from build123d import *

# Parameters (mm, degrees)
SKETCH2_W           = 33
SKETCH2_H           = 28
BOSS_EXTRUDE1_DEPTH = 46
CUT_EXTRUDE2_DEPTH  = 59.318093247
CUT_EXTRUDE4_START  = -3
CUT_EXTRUDE4_DEPTH  = 27
FILLET2_R           = 12.5
FILLET3_R           = 12.5
FILLET4_R           = 6
SKETCH7_W           = 13
SKETCH7_H           = 23
CUT_EXTRUDE5_DEPTH  = 9
SKETCH8_R           = 6.5
CUT_EXTRUDE6_DEPTH  = 9
SKETCH9_R           = 1
CUT_EXTRUDE7_DEPTH  = 9
SKETCH10_R          = 2.5
SKETCH10_R_2        = 1.3
CUT_EXTRUDE8_DEPTH  = 9


with BuildPart() as part:
    # Sketch2 → Boss-Extrude1 (new body)
    with BuildSketch(Plane.XY):
        Rectangle(SKETCH2_W, SKETCH2_H)
    extrude(amount=BOSS_EXTRUDE1_DEPTH)

    # Sketch5 → Cut-Extrude2 (cut, through all)
    with BuildSketch(Plane(origin=(16.5, 0, 0), x_dir=(0, 0, -1), z_dir=(1, 0, 0))):
        Polygon((-5, -14), (-46, 2), (-46, -14), align=None)
    extrude(amount=-CUT_EXTRUDE2_DEPTH, mode=Mode.SUBTRACT)

    # Sketch6 → Cut-Extrude4 (cut)
    with BuildSketch(Plane(origin=(16.5, 0, 0), x_dir=(0, 0, -1), z_dir=(1, 0, 0)).offset(CUT_EXTRUDE4_START)):
        Polygon((-5, -14), (-2.5, -14), (-2.5, 3.5), (-40.5, 3.5), (-40.5, -0.146341463), align=None)
    extrude(amount=-CUT_EXTRUDE4_DEPTH, mode=Mode.SUBTRACT)

    # Fillet2
    fillet2_edges = [part.edges().sort_by_distance(p)[0] for p in [
        (-13.5, 1.676829268, 40.5),
        (13.5, 1.676829268, 40.5),
    ]]
    fillet(fillet2_edges, radius=FILLET2_R)

    # Fillet3
    fillet3_edges = [part.edges().sort_by_distance(p)[0] for p in [
        (-16.5, 8, 46),
        (16.5, 8, 46),
    ]]
    fillet(fillet3_edges, radius=FILLET3_R)

    # Fillet4
    fillet4_edges = [part.edges().sort_by_distance(p)[0] for p in [
        (-16.5, -14, 2.5),
        (16.5, -14, 2.5),
    ]]
    fillet(fillet4_edges, radius=FILLET4_R)

    # Sketch7 → Cut-Extrude5 (cut)
    with BuildSketch(Plane.XZ.offset(-3.5)):
        with Locations((0, 20.5)):
            Rectangle(SKETCH7_W, SKETCH7_H)
    extrude(amount=-CUT_EXTRUDE5_DEPTH, mode=Mode.SUBTRACT)

    # Sketch8 → Cut-Extrude6 (cut)
    with BuildSketch(Plane.XZ.offset(-12.5)):
        with Locations(Location((0, 25.5, 0), (0, 0, 270))):
            Circle(SKETCH8_R)
    extrude(amount=-CUT_EXTRUDE6_DEPTH, mode=Mode.SUBTRACT)

    # Sketch9 → Cut-Extrude7 (cut)
    with BuildSketch(Plane.XZ.offset(-3.5)):
        with Locations(Location((0, 34.3, 0), (0, 0, 270))):
            Circle(SKETCH9_R)
        with Locations(Location((0, 6.7, 0), (0, 0, 270))):
            Circle(SKETCH9_R)
    extrude(amount=-CUT_EXTRUDE7_DEPTH, mode=Mode.SUBTRACT)

    # Sketch10 → Cut-Extrude8 (cut)
    with BuildSketch(Plane(origin=(0, 0, 0), x_dir=(-1, 0, 0), z_dir=(0, 0, -1))):
        with Locations((-5, 0)):
            Circle(SKETCH10_R)
        with Locations((-0.5, 0)):
            Circle(SKETCH10_R_2)
        with Locations((-9.5, 0)):
            Circle(SKETCH10_R_2)
    extrude(amount=-CUT_EXTRUDE8_DEPTH, mode=Mode.SUBTRACT)


solid = part.part
Check sheet for the modelled part. Datum: model origin and axes. Units: mm. A direction names the side the tool comes from. Round coordinates to 2 decimals unless told otherwise and drop trailing zeros. Order: outer loops, then holes, each group sorted by start corner. A loop starts at its lowest first (then second) coordinate and runs counter-clockwise, first axis right, second up.
(1) Cross-section at B-B, the plane y = 11.25. Enter the section's corners in (x, z), and give its area (3 significant figures).
(2) Scan lines: probe 1 along X at (y, z) = (2.5, 12.5); probe 2 along Y at (x, z) = (9.5, 1.4); probe 3 along X at (y, z) = (9, 6.7). Record each from-to range of solid material in increasing order.
(3) Go/stop test with flat-tipped pins: P1, Ø7, axis at x = -2, z = 29, coming from the -Y side; P2, Ø2, axis at x = 0.5, y = 0, coming from the -Z side; P3, Ø0.6, axis at x = 0, z = 7, coming from the -Y side; P4, Ø11.5, axis at x = 0, z = 25.5, coming from the -Y side. Record where each tip stops, or that it passes through.
(4) Access from +Z, -Z, +X, -X, +Y, -Y to the whole of each face (thin tool, end or side, straight path). Record for faces 4 (the cylindrical face through (0.67, 1.29, 1.23)), 5 (the cylindrical face through (15.91, -10.595, 5.802)), 6 (the flat face through (0, 12.5, 34)).
(5) Cross-section at A-A, the plane x = 5. Enter the section's corners in (y, z).
(6) Cross-section at C-C, the plane x = -2. Enter the section's corners in (y, z).
(7) Cross-section at D-D, the plane z = 38.5. Enter the section's corners in (x, y), and give its area (3 significant figures).
(8) Draft check along Z on faces 1 (the cylindrical face through (-12.935, 7.554, 42.241)), 2 (the flat face through (0, 12.5, 14)), 3 (the flat face through (-16.5, 3, 17)). Enter one of: pulls with the +Z half, pulls with the -Z half, needs draft (parallel to the pull), parting line crosses it, or undercut.
Check sheet entries:
1. outline: (-16.5, 0) - (16.5, 0) - (16.5, 33.5) arc R12.5 ccw to (4, 46) - (-4, 46) arc R12.5 ccw to (-16.5, 33.5) - close; hole (-6.5, 9) - (6.5, 9) - (6.5, 32) - (-6.5, 32) - close; hole circle Ø2 at (0, 6.7); hole circle Ø2 at (0, 34.3)
1. area: 1,150 mm2
2. probe 1: x = -16.5 to -13.5, 13.5 to 16.5
2. probe 2: y = -14 to -1.3, 1.3 to 14
2. probe 3: x = -16.5 to -1, 1 to 16.5
3. P1: stops at y = 3.5
3. P2: stops at z = 40.49
3. P3: stops at y = 12.5
3. P4: passes through
4. face 4: -Z
4. face 5: +Z, -Z, +X, -Y
4. face 6: -Y
5. outline: (-14, 0) - (-2.5, 0) - (-2.5, 2.5) - (-14, 2.5) - close; (-0.4, 39.84) - (3.5, 39.84) - (3.5, 32) - (12.5, 32) - (12.5, 29.65) - (14, 29.65) - (14, 45.96) - (1.98, 45.96) - close; (2.5, 0) - (14, 0) - (14, 21.35) - (12.5, 21.35) - (12.5, 9) - (3.5, 9) - (3.5, 2.5) - (2.5, 2.5) - close
6. outline: (-14, 0) - (14, 0) - (14, 19.32) - (12.5, 19.32) - (12.5, 9) - (3.5, 9) - (3.5, 2.5) - (-14, 2.5) - close; (-0.16, 40.46) - (3.5, 40.46) - (3.5, 32) - (12.5, 32) - (12.5, 31.68) - (14, 31.68) - (14, 46) - (2, 46) - close
7. outline: (-15.46, -0.93) - (-7.78, -0.93) - (-7.78, 3.5) - (7.78, 3.5) - (7.78, -0.93) - (15.46, -0.93) - (15.46, 14) - (-15.46, 14) - close
7. area: 393 mm2
8. face 1: pulls with the +Z half
8. face 2: undercut
8. face 3: needs draft
